Autodesk Inventor part; units mm, degrees
ref_plane "YZ Plane" through (0, 0, 0) normal (1, 0, 0) x (0, 1, 0)
ref_plane "XZ Plane" through (0, 0, 0) normal (0, 1, 0) x (-1, 0, 0)
ref_plane "XY Plane" through (0, 0, 0) normal (0, 0, 1) x (1, 0, 0)
sketch "Sketch1" plane through (0, 0, 0) normal (1, 0, 0) x (0, 1, 0)
  line L0 (0, 0) -> (25, 0)
  line L1 (25, 0) -> (25, -125)
  line L2 (25, -125) -> (0, -125)
  line L3 (0, -125) -> (0, -123)
  line L4 (0, -123) -> (23, -123)
  line L5 (23, -123) -> (23, -2)
  line L6 (23, -2) -> (0, -2)
  line L7 (0, -2) -> (0, 0)
  dimension "d0" = 2
  dimension "d1" = 2
  dimension "d2" = 125
  dimension "d3" = 25
  dimension "d4" = 2
extrude "Extrusion1" add sketch "Sketch1" along normal blind 200 and the other way blind 70
sketch "Sketch2" plane through (-70, 25, 0) normal (0, 1, 0) x (1, 0, 0)
  circle A0 centre (80, 22) radius 2.75
  circle A1 centre (80, 47) radius 2.75
  circle A2 centre (110, 22) radius 2.75
  circle A3 centre (110, 47) radius 2.75
  line L0 (0, 0) -> (0, 125)
  line L1 (270, 0) -> (0, 0)
  circle A4 centre (9.057, 101.86) radius 2.65
  circle A5 centre (9.057, 87.86) radius 2.65
  circle A6 centre (39.057, 101.86) radius 2.65
  circle A7 centre (39.057, 87.86) radius 2.65
  line L2 (270, 125) -> (0, 125)
  point P0 (70, 0)
  dimension "d9" = 5.5
  dimension "d10" = 5.5
  dimension "d11" = 5.5
  dimension "d12" = 5.5
  dimension "d13" = 80
  dimension "d14" = 80
  dimension "d15" = 22
  dimension "d16" = 110
  dimension "d17" = 110
  dimension "d18" = 22
  dimension "d19" = 25
  dimension "d20" = 25
  dimension "d23" = 5.3
  dimension "d24" = 5.3
  dimension "d25" = 5.3
  dimension "d26" = 5.3
  dimension "d27" = 9.057
  dimension "d28" = 9.057
  dimension "d29" = 14
  dimension "d30" = 30
  dimension "d31" = 30
  dimension "d32" = 14
  dimension "d33" = 30
  dimension "d34" = 14
  dimension "d36" = 23.14
extrude "Extrusion2" cut sketch "Sketch2" against normal blind 10
sketch "Sketch3" plane through (-70, 0, 0) normal (0, 0, 1) x (1, 0, 0)
  circle A0 centre (80, 12.5) radius 2.75
  line L0 (0, 0) -> (270, 0)
  line L1 (0, 0) -> (0, 25)
  circle A1 centre (257.5, 12.5) radius 2.75
  line L2 (270, 25) -> (0, 25)
  line L3 (270, 25) -> (270, 0)
  point P0 (70, 0)
  dimension "d37" = 5.5
  dimension "d38" = 12.5
  dimension "d39" = 80
  dimension "d40" = 5.5
  dimension "d41" = 12.5
  dimension "d42" = 12.5
extrude "Extrusion3" cut sketch "Sketch3" against normal blind 142 contours A0 | A1
properties part number "Spacer Extrusion" material "Aluminum 6061"
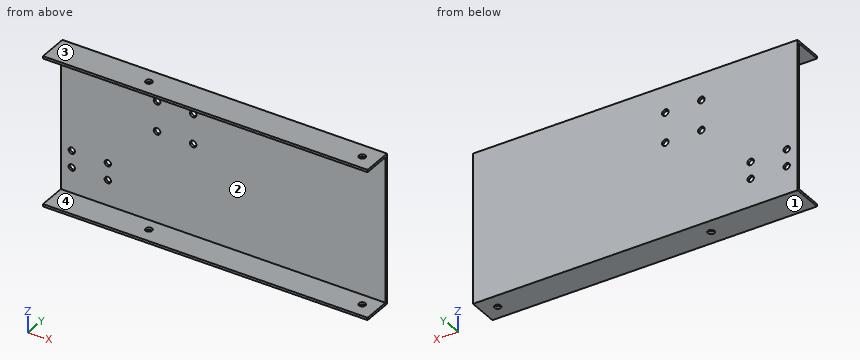
Source: CAD feature listing. Evaluate the final solid. Frame: model axes, mm. Face numbers are marked on the shaded views. Coordinates: 2 decimals unless noted, no trailing zeros. Write each loop counter-clockwise with the first axis right and the second up, starting at its lowest first coordinate (ties: lowest second). Pieces come first, ordered by that corner, then holes. Notation, with made-up numbers: (26, 49.5) -> (67, 49.5) arc R17 cw to (67, 76.5) -> close; hole circle Ø6 at (3.5, 70). An arc over 180 degrees is marked (long way). Return JSON: item names as keys, results as strings. Group by question number.
1) Section query C-C, the plane z = -87.86. Return loops of the section in (x, y), plus the area to 3 significant figures.
2) Mould query, pull axis Z, two halves, no side actions, for the marked faces 1, 2, 3 and 4. Classes: +Z half, -Z half, draft (parallel to the pull), parting line (faces both ways), or undercut.
3) Section query B-B, the plane y = 5. Return loops of the section in (x, z).
4) Contact query for flat-ended pins moving along their axis: P1, Ø5, axis at x = -25, z = -66, coming from the -Y side; P2, Ø5, axis at x = 10, z = -22, coming from the +Y side. Output: stop coordinate, or through.
5) Section query A-A, the plane x = 40. Return loops of the section in (y, z), plus the area to 3 significant figures.
6) Ray query, line 1 along X through (y, z) = (23.8, -87.86); line 2 along Z through (x, y) = (154, 14); line 3 along X through (y, z) = (24.4, -22). Return the intervals inside material, ascending.
7) Section query D-D, the plane x = 10. Return loops of the section in (y, z), plus the area to 3 significant figures.
From the geometry:
{
 "1": {"outline": "(-70, 23) -> (-63.59, 23) -> (-63.59, 25) -> (-70, 25) -> close; (-58.29, 23) -> (-33.59, 23) -> (-33.59, 25) -> (-58.29, 25) -> close; (-28.29, 23) -> (200, 23) -> (200, 25) -> (-28.29, 25) -> close", "area": "519 mm²"},
 "2": {"face 1": "-Z half", "face 2": "undercut", "face 3": "+Z half", "face 4": "undercut"},
 "3": {"outline": "(-70, -125) -> (200, -125) -> (200, -123) -> (-70, -123) -> close; (-70, -2) -> (200, -2) -> (200, 0) -> (-70, 0) -> close"},
 "4": {"P1": "y = 23", "P2": "through"},
 "5": {"outline": "(0, -125) -> (25, -125) -> (25, -49.75) -> (23, -49.75) -> (23, -123) -> (0, -123) -> close; (0, -2) -> (23, -2) -> (23, -19.25) -> (25, -19.25) -> (25, 0) -> (0, 0) -> close; (23, -44.25) -> (25, -44.25) -> (25, -24.75) -> (23, -24.75) -> close", "area": "320 mm²"},
 "6": {"line 1": "-70 to -63.59, -58.29 to -33.59, -28.29 to 200", "line 2": "-125 to -123, -2 to 0", "line 3": "-70 to 7.25, 12.75 to 37.25, 42.75 to 200"},
 "7": {"outline": "(0, -125) -> (9.75, -125) -> (9.75, -123) -> (0, -123) -> close; (0, -2) -> (9.75, -2) -> (9.75, 0) -> (0, 0) -> close; (15.25, -125) -> (25, -125) -> (25, -49.75) -> (23, -49.75) -> (23, -123) -> (15.25, -123) -> close; (15.25, -2) -> (23, -2) -> (23, -19.25) -> (25, -19.25) -> (25, 0) -> (15.25, 0) -> close; (23, -44.25) -> (25, -44.25) -> (25, -24.75) -> (23, -24.75) -> close", "area": "298 mm²"}
}
